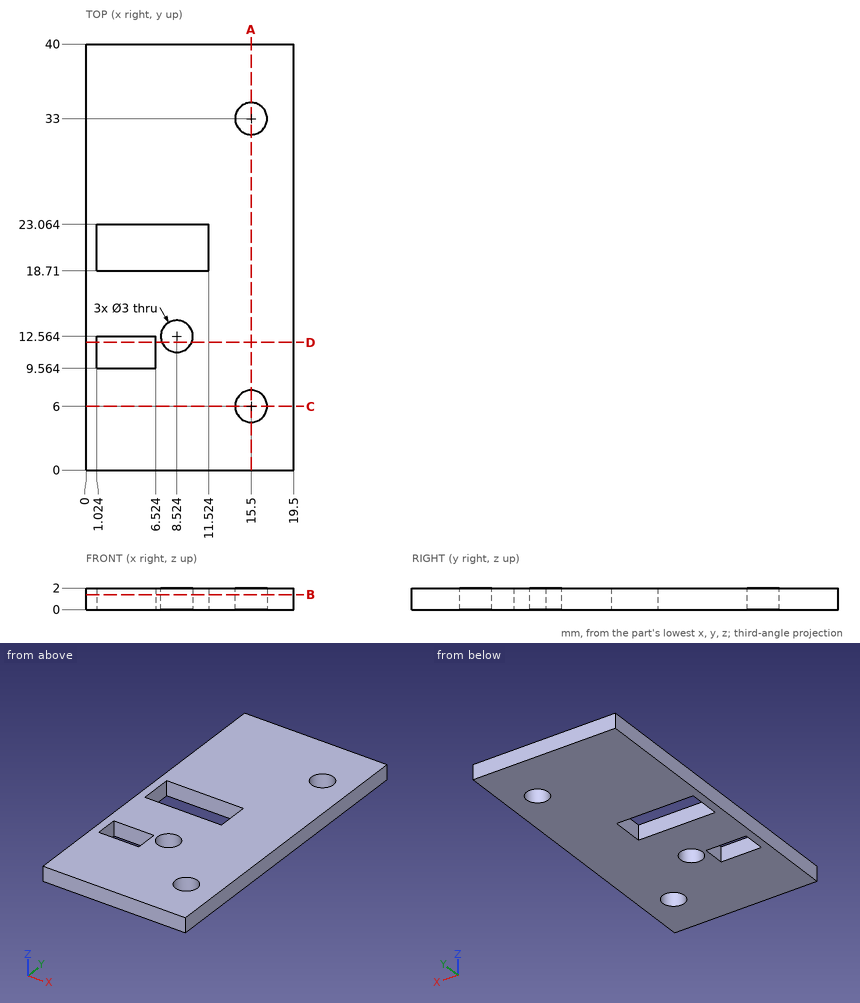
Can you work these out from the drawing? Everything is in mm from the part's minimum corner. Give positions to 0.01 mm unless a question says otherwise; leave off trailing zeros. Order: outer loops, then holes, each group sorted by start corner. A loop starts at its lowest first (then second) coordinate and runs counter-clockwise, first axis right, second up. Notation, with made-up numbers: M 13.25,52 L 28.25,52 A16 cw 28.25,69 Z; hole C 66.5,57.25 d4. An arc over 180 degrees is marked long. Use a Markdown table: item, result. Add a question column.
Item 1: Suppose I cut it at C-C (y = 6). List the corners of the cut face in (x, z) for me.
Item 2: Suppose I cut it at A-A (x = 15.5). List the corners of the cut face in (y, z) for me.
Item 3: Suppose I cut it at B-B (z = 1.4). List the corners of the cut face in (x, y) for me.
Item 4: Will this pin go through, and if not, where does the flat tip stop? pin 1 (0.6 mm diameter, centred on y = 10.5, z = 1.5, fed in from -X).
Item 5: Suppose I cut it at D-D (y = 12). List the corners of the cut face in (x, z) for me.
Item 6: If I drill on L1, parallel to Y at x = 15.5, z = 1.35; L2, parallel to Y at x = 6, z = 1.4; L3, parallel to X at y = 10.5, z = 0.9, over which ranges is the centre line in solid material (lowest first)? Write a range as [from, to].
Answer sheet:
| question | item | result |
|---|---|---|
| 1 | outline | M 0,0 L 14,0 L 14,2 L 0,2 Z; M 17,0 L 19.5,0 L 19.5,2 L 17,2 Z |
| 2 | outline | M 0,0 L 4.5,0 L 4.5,2 L 0,2 Z; M 7.5,0 L 31.5,0 L 31.5,2 L 7.5,2 Z; M 34.5,0 L 40,0 L 40,2 L 34.5,2 Z |
| 3 | outline | M 0,0 L 19.5,0 L 19.5,40 L 0,40 Z; hole M 1.02,9.56 L 6.52,9.56 L 6.52,12.56 L 1.02,12.56 Z; hole M 1.02,18.71 L 11.52,18.71 L 11.52,23.06 L 1.02,23.06 Z; hole C 8.52,12.56 d3; hole C 15.5,6 d3; hole C 15.5,33 d3 |
| 4 | pin 1 | stops at x = 0 |
| 5 | outline | M 0,0 L 1.02,0 L 1.02,2 L 0,2 Z; M 6.52,0 L 7.13,0 L 7.13,2 L 6.52,2 Z; M 9.91,0 L 19.5,0 L 19.5,2 L 9.91,2 Z |
| 6 | L1 | y = [0, 4.5], [7.5, 31.5], [34.5, 40] |
| 6 | L2 | y = [0, 9.56], [12.56, 18.71], [23.06, 40] |
| 6 | L3 | x = [0, 1.02], [6.52, 19.5] |
